Verification items for the finished model (mm, model axes). A direction names the side the tool comes from. Give positions to 0.01 mm unless a question says otherwise; leave off trailing zeros. Write each loop counter-clockwise with the first axis right and the second up, starting at its lowest first coordinate (ties: lowest second). Pieces come first, ordered by that corner, then holes. Notation, with made-up numbers: (37, -30) -> (71, -30) arc R17 cw to (71, -23) -> close; hole circle Ø4 at (-14.75, 21.25). An arc over 180 degrees is marked (long way). Use one line per item in the form item = value. Start each with the question number.
(1) Release check for a two-part mould opening along Z. For faces 4 (the face through (3.5, 1.3, 31.8)), 5 (the face through (0, 2.5, -1)), 6 (the face through (3.467, 1.264, -31.693)) record: pulls with the +Z half, pulls with the -Z half, needs draft (parallel to the pull), parting line crosses it, or undercut.
(2) Section check C-C, the plane z = 6. Record the cut outline in (x, y).
(3) Set-up check for faces 1 (the face through (3, 1, 0)), 2 (the face through (-3, 1, 0)), 3 (the face through (0, 1, 44)): record each of +Z, -Z, +X, -X, +Y, -Y from which the full face is reachable in a straight line by a thin tool's end or side.
(4) Depth check by flat-ended pin: pin 1 Ø2.5 at (x, z) = (0, 38) entering from -Y. Enter the tip coordinate at first touch or a pass-through.
(5) Section check A-A, the plane x = 0. Record the cut outline in (y, z), plus the area to 3 significant figures.
(6) Section check B-B, the plane y = 1.1. Record the cut outline in (x, z) (3 decimals), plus the area to 3 significant figures.
(7) Scan lines: L1, parallel to Z at x = 0, y = 1.15; L2, parallel to X at y = 0.85, z = 38; L3, parallel to X at y = 2.2, z = 27. Record each from-to range of solid material in increasing order.
from build123d import *

# Parameters (mm, degrees)
SKETCH1_R           = 2
BOSS_EXTRUDE1_DEPTH = 2.5
FILLET1_R           = 10
FILLET2_R           = 0.25


with BuildPart() as part:
    # Sketch1 → Boss-Extrude1 (new body)
    with BuildSketch(Plane(origin=(0, 0, 0), x_dir=(1, 0, 0), z_dir=(0, 1, 0))):
        with BuildLine():
            ThreePointArc((-3, -32.803847577), (0, -44), (3, -32.803847577))
            Line((3, -32.803847577), (3, 32.803847577))
            ThreePointArc((3, 32.803847577), (0, 44), (-3, 32.803847577))
            Line((-3, 32.803847577), (-3, -32.803847577))
        make_face()
        with Locations((0, -38)):
            Circle(SKETCH1_R, mode=Mode.SUBTRACT)
        with Locations((0, 38)):
            Circle(SKETCH1_R, mode=Mode.SUBTRACT)
    extrude(amount=BOSS_EXTRUDE1_DEPTH)

    # Fillet1
    fillet1_edges = [part.edges().sort_by_distance(p)[0] for p in [
        (-3, 1.25, 32.803847577),
        (-3, 1.25, -32.803847577),
        (3, 1.25, -32.803847577),
        (3, 1.25, 32.803847577),
    ]]
    fillet(fillet1_edges, radius=FILLET1_R)

    # Fillet2
    fillet2_edges = [part.edges().sort_by_distance(p)[0] for p in [
        (0, 0, 44),
        (0, 2.5, 44),
        (-3, 0, 0),
        (-3, 2.5, 0),
        (0, 0, -44),
        (0, 2.5, -44),
        (3, 0, 0),
        (3, 2.5, 0),
        (-3.480283618, 0, 31.734483125),
        (-3.480283618, 2.5, 31.734483125),
        (-3.480283618, 0, -31.734483125),
        (-3.480283618, 2.5, -31.734483125),
        (3.480283618, 0, -31.734483125),
        (3.480283618, 2.5, -31.734483125),
        (3.480283618, 0, 31.734483125),
        (3.480283618, 2.5, 31.734483125),
    ]]
    fillet(fillet2_edges, radius=FILLET2_R)


solid = part.part
Completed:
q1.face_4 = undercut
q1.face_5 = needs draft
q1.face_6 = undercut
q2.outline = (-3, 0.25) arc R0.25 ccw to (-2.75, 0) -> (2.75, 0) arc R0.25 ccw to (3, 0.25) -> (3, 2.25) arc R0.25 ccw to (2.75, 2.5) -> (-2.75, 2.5) arc R0.25 ccw to (-3, 2.25) -> close
q3.face_1 = +X, +Y, -Y
q3.face_2 = -X, +Y, -Y
q3.face_3 = +Y, -Y
q4.pin_1 = through
q5.outline = (0, -43.75) arc R0.25 ccw to (0.25, -44) -> (2.25, -44) arc R0.25 ccw to (2.5, -43.75) -> (2.5, -40) -> (0, -40) -> close; (0, -36) -> (2.5, -36) -> (2.5, 36) -> (0, 36) -> close; (0, 40) -> (2.5, 40) -> (2.5, 43.75) arc R0.25 ccw to (2.25, 44) -> (0.25, 44) arc R0.25 ccw to (0, 43.75) -> close
q5.area = 200 mm²
q6.outline = (-4.875, -34.502) arc R6 ccw (long way) to (4.875, -34.502) arc R10 cw to (3, -28.673) -> (3, 28.673) arc R10 cw to (4.875, 34.502) arc R6 ccw (long way) to (-4.875, 34.502) arc R10 cw to (-3, 28.673) -> (-3, -28.673) arc R10 cw to start; hole circle Ø4 at (0, -38); hole circle Ø4 at (0, 38)
q6.area = 595 mm²
q7.L1 = -44 to -40, -36 to 36, 40 to 44
q7.L2 = -6 to -2, 2 to 6
q7.L3 = -3 to 3
